```python
from build123d import *

# Parameters (mm, degrees)
SKETCH_1_R      = 1.7
EXTRUDE_1_DEPTH = 4
EXTRUDE_START   = -8
EXTRUDE_2_DEPTH = 8


with BuildPart() as part:
    # Эскиз1 → Бобышка-Вытянуть1 (new body)
    with BuildSketch(Plane(origin=(0, 0, 0), x_dir=(1, 0, 0), z_dir=(0, 1, 0))):
        with BuildLine():
            Line((0, -50), (0, -43))
            add(Edge.make_bspline(
                [(-10.000145873, 27.475174978), (-27.697978685, -43), (0, -43)],
                knots=[4.019246634, 4.019246634, 4.019246634, 6.283185307, 6.283185307, 6.283185307], degree=2, weights=[1, 0.42487789, 1]))
            ThreePointArc((-10.000145873, 27.475174978), (-18.360814479, 27.113576543), (-26.230013338, 24.266254592))
            add(Edge.make_bspline(
                [(-26.230013338, 24.266254592), (-50.964235719, -50), (0, -50)],
                knots=[4.205654034, 4.205654034, 4.205654034, 6.283185307, 6.283185307, 6.283185307], degree=2, weights=[1, 0.507284392, 1]))
        make_face()
        with Locations(Location((-3.997292475, -45.689262056, 0), (0, 0, 270))):
            Circle(SKETCH_1_R, mode=Mode.SUBTRACT)
        with Locations(Location((-21.5, 0, 0), (0, 0, 270))):
            Circle(SKETCH_1_R, mode=Mode.SUBTRACT)
    extrude(amount=EXTRUDE_1_DEPTH)

    # Эскиз2 → Бобышка-Вытянуть2 (add)
    with BuildSketch(Plane(origin=(0, 4, 0), x_dir=(1, 0, 0), z_dir=(0, 1, 0)).offset(EXTRUDE_START)):
        with BuildLine():
            Line((0, -43), (0, -38))
            add(Edge.make_bspline(
                [(-6.021112225, 26.742839981), (-29.868438829, -38), (0, -38)],
                knots=[3.78773541, 3.78773541, 3.78773541, 6.283185307, 6.283185307, 6.283185307], degree=2, weights=[1, 0.317480533, 1]))
            ThreePointArc((-6.021112225, 26.742839981), (-8.200317768, 27.218512364), (-10.410783781, 27.516909787))
            add(Edge.make_bspline(
                [(-10.410783781, 27.516909787), (-37.171364773, -43), (0, -43)],
                knots=[3.908695263, 3.908695263, 3.908695263, 6.283185307, 6.283185307, 6.283185307], degree=2, weights=[1, 0.374216095, 1]))
        make_face()
    extrude(amount=EXTRUDE_2_DEPTH)


solid = part.part
```
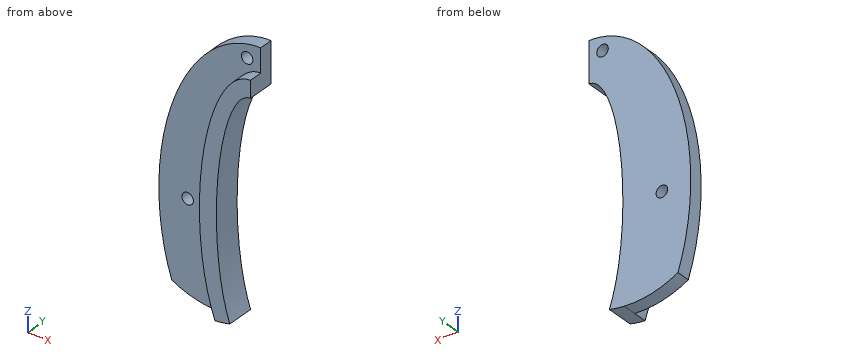
For this review, take the finished solid that the model builds, in its own axes (mm). Round coordinates to 2 decimals unless told otherwise and drop trailing zeros. Answer as CSV lines item,"result". Start each with the question number.
(1) For pin 1 (2 mm diameter, centred on y = 0.5, z = 25.5, fed in from +X); pin 2 (5.5 mm diameter, centred on x = -21.5, z = 0, fed in from +Y), all flat-tipped, find the tip position at first contact; note any pin that passes through.
(2) Add section A-A, the plane y = 1. State how many separate pieces and enclosed holes the cut face has, plus the area to 3 significant figures.
(3) For line 1 (X direction, y = 0.95, z = 0); line 2 (Y direction, x = -16, z = 38.5); line 3 (X direction, y = -1.25, z = 1), list the stretches that pass through material, from the lowest coordinate up.
From the geometry:
1,pin 1,"stops at x = -7.33"
1,pin 2,"stops at y = 4"
2,separate pieces,"1"
2,enclosed holes,"2"
2,area,"1,390 mm²"
3,line 1,"x = -30 to -23.2, -19.8 to -9.98"
3,line 2,"y = 0 to 4"
3,line 3,"x = -15 to -10"
